The figure shows three views and two pictorial views of one solid part (mm, origin at its lowest corner). Answer the questions. Round coordinates to 2 decimals unless told otherwise and drop trailing zeros. Write each loop counter-clockwise with the first axis right and the second up, starting at its lowest first coordinate (ties: lowest second). Pieces come first, ordered by that corner, then holes. Notation, with made-up numbers: M 0,29 L 20,29 A35 cw 20,64 Z; hole C 33,61 d9. An arc over 180 degrees is marked long. Answer in a Markdown table with one row per item.
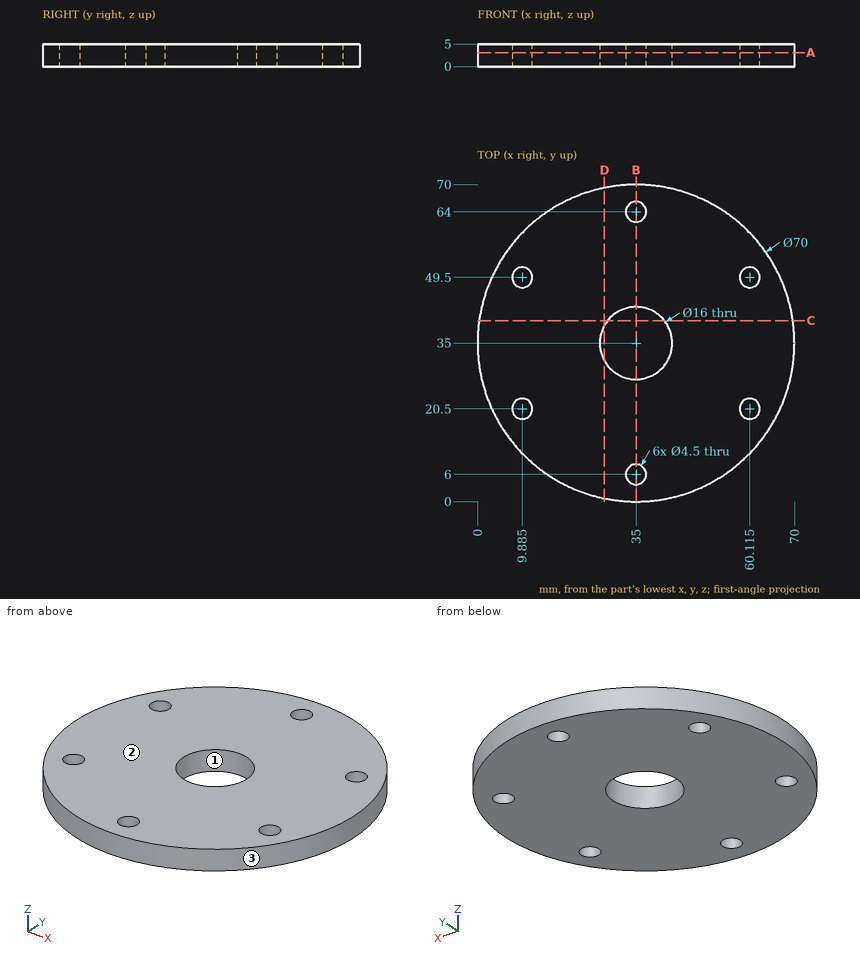
1. The part is cut by section A-A (z = 3.1). Count the separate pieces of the cut face and the enclosed holes in it, plus the area to 3 significant figures.
Calculated:
| item | result |
|---|---|
| separate pieces | 1 |
| enclosed holes | 7 |
| area | 3,550 mm² |
2. Given pin 1 (5 mm diameter, centred on x = 9.89, y = 49.5, fed in from -Z); pin 2 (2 mm diameter, centred on y = 20, z = 1, fed in from -X); pin 3 (1 mm diameter, centred on x = 20.5, z = 0.5, fed in from -Y), each flat-ended and moving along its own axis, determine where each tip first touches the part or whether it passes through.
Calculated:
| item | result |
|---|---|
| pin 1 | stops at z = 0 |
| pin 2 | stops at x = 2.92 |
| pin 3 | stops at y = 2.92 |
3. The part is cut by section B-B (x = 35). Determine the outline of the cut face in (y, z), plus the area to 3 significant figures.
Calculated:
| item | result |
|---|---|
| outline | M 0,0 L 3.75,0 L 3.75,5 L 0,5 Z; M 8.25,0 L 27,0 L 27,5 L 8.25,5 Z; M 43,0 L 61.75,0 L 61.75,5 L 43,5 Z; M 66.25,0 L 70,0 L 70,5 L 66.25,5 Z |
| area | 225 mm² |
4. Consider line 1 along Y through (x, z) = (35, 3.7); line 2 along Y through (x, z) = (36, 1.6) (1 decimal); line 3 along Y through (x, z) = (41, 3.85). Determine where each line is inside the solid, lowest interval first. Write a range as from..to.
Calculated:
| item | result |
|---|---|
| line 1 | y = 0..3.75, 8.25..27, 43..61.75, 66.25..70 |
| line 2 | y = 0..4, 8..27.1, 42.9..62, 66..70 |
| line 3 | y = 0.52..29.71, 40.29..69.48 |
5. Determine the mould class of the marked faces 1, 2 and 3 for opening direction Y: released by +Y, released by -Y, zero draft, split by the parting line, or undercut.
Calculated:
| item | result |
|---|---|
| face 1 | undercut |
| face 2 | zero draft |
| face 3 | split by the parting line |
6. The part is cut by section D-D (x = 28). Determine the outline of the cut face in (y, z).
Calculated:
| item | result |
|---|---|
| outline | M 0.71,0 L 31.13,0 L 31.13,5 L 0.71,5 Z; M 38.87,0 L 69.29,0 L 69.29,5 L 38.87,5 Z |
7. The part is cut by section C-C (y = 40). Determine the outline of the cut face in (x, z) (1 decimal).
Calculated:
| item | result |
|---|---|
| outline | M 0.4,0 L 28.8,0 L 28.8,5 L 0.4,5 Z; M 41.2,0 L 69.6,0 L 69.6,5 L 41.2,5 Z |
